Source: CAD feature listing. Evaluate the final solid. Frame: model axes, mm. Face numbers are marked on the shaded views. A direction names the side the tool comes from. Coordinates: 2 decimals unless noted, no trailing zeros. Order: outer loops, then holes, each group sorted by start corner. A loop starts at its lowest first (then second) coordinate and runs counter-clockwise, first axis right, second up. Notation, with made-up numbers: (24.5, 1.25) - (75.5, 1.25) arc R6 cw to (75.5, 6.25) - close; hole circle Ø3 at (26, 49.25). An arc over 180 degrees is marked (long way). One line per question, with ' | ' between items. Start each with the question number.
(1) Section B-B (z = 10). Return the cut outline in (x, y) (3 decimals).
(2) Access query for the marked faces 1, 2 and 3. Directions: +Z, -Z, +X, -X, +Y, -Y. A direction counts if a zero-diameter tool reaches every point of the face in a straight line with its end or side. Return the directions, or none.
(3) Draft query along X for the marked faces 4, 5 and 6. Return one class per face: +X half, -X half, draft (parallel to the pull), parting line (faces both ways), or undercut.
(4) Section A-A (x = 15). Return the cut outline in (y, z) (3 decimals).
(5) Contact query for flat-ended pins moving along their axis: P1, Ø3, axis at x = 16, z = 20.5, coming from the -Y side; P2, Ø6, axis at x = 26.5, y = -4.5, coming from the +Z side. Output: stop coordinate, or through.
(6) Line query: line 1 along Z through (x, y) = (15, -7); line 2 along Z through (x, y) = (1.5, -8.75); line 3 along X through (y, z) = (-10.5, 18.5). Output: solid intervals per line, ascending.
(7) Section C-C (y = -20). Return the cut outline in (x, z) (3 decimals), then the cut area to 3 significant figures.
(8) Section D-D (y = -8). Return the cut outline in (x, z), then the cut area to 3 significant figures.
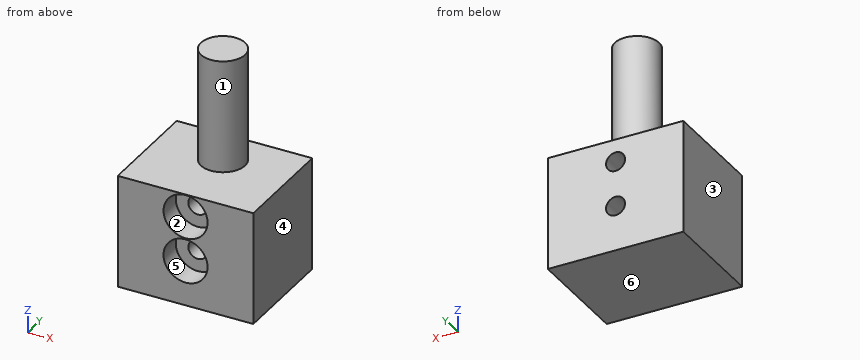
from build123d import *

# Parameters (mm, degrees)
F0_W           = 30
F0_H           = 24
F1_DEPTH       = 25
F3_D           = 4.2
F3_CBORE_D     = 9.75
F3_CBORE_DEPTH = 5
F4_R           = 4.8868240238
F5_DEPTH       = 25


with BuildPart() as f1:
    # F0 (on Top) → F1 (new body)
    with BuildSketch(Plane.XY):
        with Locations((15, -12)):
            Rectangle(F0_W, F0_H)
    extrude(amount=F1_DEPTH)

    # F3 (through all)
    with Locations(Plane.XZ.offset(24)):
        with Locations((15, 20), (15, 10)):
            CounterBoreHole(F3_D / 2, F3_CBORE_D / 2, F3_CBORE_DEPTH)

    # F4 (on face) → F5 (join)
    with BuildSketch(Plane.XY.offset(25)):
        with Locations((15, -8.7359920144)):
            Circle(F4_R)
    extrude(amount=F5_DEPTH)


solid = f1.part
Response values:
1) outline: (0, -24) - (10.125, -24) - (10.125, -19) - (12.9, -19) - (12.9, 0) - (0, 0) - close; (17.1, -19) - (19.875, -19) - (19.875, -24) - (30, -24) - (30, 0) - (17.1, 0) - close
2) face 1: +Z | face 2: -Y | face 3: +Z, -Z, -X, +Y, -Y
3) face 4: +X half | face 5: undercut | face 6: draft
4) outline: (-24, 0) - (0, 0) - (0, 7.9) - (-19, 7.9) - (-19, 5.125) - (-24, 5.125) - close; (-24, 14.875) - (-19, 14.875) - (-19, 12.1) - (0, 12.1) - (0, 17.9) - (-19, 17.9) - (-19, 15.125) - (-24, 15.125) - close; (-24, 24.875) - (-19, 24.875) - (-19, 22.1) - (0, 22.1) - (0, 25) - (-3.849, 25) - (-3.849, 50) - (-13.623, 50) - (-13.623, 25) - (-24, 25) - close
5) P1: stops at y = -19 | P2: stops at z = 25
6) line 1: z = 0 to 7.9, 12.1 to 17.9, 22.1 to 50 | line 2: z = 0 to 25 | line 3: x = 0 to 13.53, 16.47 to 30
7) outline: (0, 0) - (30, 0) - (30, 25) - (0, 25) - close; hole circle Ø9.75 at (15, 10); hole circle Ø9.75 at (15, 20) | area: 601 mm²
8) outline: (0, 0) - (30, 0) - (30, 25) - (19.83, 25) - (19.83, 50) - (10.17, 50) - (10.17, 25) - (0, 25) - close; hole circle Ø4.2 at (15, 10); hole circle Ø4.2 at (15, 20) | area: 964 mm²
